Input: part model. Units: mm. Frame: model coordinates. A direction names the side the tool comes from. Round coordinates to 2 decimals unless told otherwise and drop trailing zeros. Order: outer loops, then holes, each group sorted by start corner. A loop starts at its lowest first (then second) coordinate and runs counter-clockwise, first axis right, second up. Notation, with made-up numbers: (76.5, 27) -> (94.5, 27) arc R14 ccw to (94.5, 34) -> close; hole circle Ø9 at (55.5, 30.25). An arc over 180 degrees is marked (long way). Use a Markdown table: item, result.
from build123d import *

# Parameters (mm, degrees)
SKETCH1_W                                       = 15
SKETCH1_H                                       = 24
BOSS_EXTRUDE1_DEPTH                             = 3
SKETCH2_W                                       = 8
SKETCH2_H                                       = 5
BOSS_EXTRUDE2_DEPTH                             = 6
CSK_FOR_M2_FLAT_HEAD_MACHINE_SCREW1_D           = 2.4
CSK_FOR_M2_FLAT_HEAD_MACHINE_SCREW1_CSINK_D     = 4.4
CSK_FOR_M2_FLAT_HEAD_MACHINE_SCREW1_CSINK_ANGLE = 90
FILLET1_R                                       = 2
SKETCH5_R                                       = 1.5
CUT_EXTRUDE1_DEPTH                              = 3
FILLET2_R                                       = 4


with BuildPart() as part:
    # Sketch1 → Boss-Extrude1 (new body)
    with BuildSketch(Plane.XY):
        Rectangle(SKETCH1_W, SKETCH1_H)
    extrude(amount=BOSS_EXTRUDE1_DEPTH)

    # Sketch2 → Boss-Extrude2 (add)
    with BuildSketch(Plane.XY.offset(3)):
        with Locations((0, -9.5)):
            Rectangle(SKETCH2_W, SKETCH2_H)
    extrude(amount=BOSS_EXTRUDE2_DEPTH)

    # CSK for M2 Flat Head Machine Screw1 (through all)
    with Locations(Plane(origin=(0, -7, 6), x_dir=(0, 0, 1), z_dir=(0, 1, 0))):
        with Locations((0, 0)):
            CounterSinkHole(CSK_FOR_M2_FLAT_HEAD_MACHINE_SCREW1_D / 2, CSK_FOR_M2_FLAT_HEAD_MACHINE_SCREW1_CSINK_D / 2, counter_sink_angle=CSK_FOR_M2_FLAT_HEAD_MACHINE_SCREW1_CSINK_ANGLE)

    # Fillet1
    fillet1_edges = [part.edges().sort_by_distance(p)[0] for p in [
        (-4, -9.5, 9),
        (4, -9.5, 9),
    ]]
    fillet(fillet1_edges, radius=FILLET1_R)

    # Sketch5 → Cut-Extrude1 (cut)
    with BuildSketch(Plane(origin=(0, 0, 0), x_dir=(-1, 0, 0), z_dir=(0, 0, -1))):
        with Locations((0, 5.5)):
            Circle(SKETCH5_R)
    extrude(amount=-CUT_EXTRUDE1_DEPTH, mode=Mode.SUBTRACT)

    # Fillet2
    fillet2_edges = [part.edges().sort_by_distance(p)[0] for p in [
        (-7.5, 12, 1.5),
        (7.5, 12, 1.5),
    ]]
    fillet(fillet2_edges, radius=FILLET2_R)


solid = part.part
1) Ray query, probe 1 along Z at (x, y) = (0, -10.5); probe 2 along X at (y, z) = (-10.3, 6); probe 3 along Y at (x, z) = (0, 1.1). Return the intervals inside material, ascending.
Answer key:
| item | result |
|---|---|
| probe 1 | z = 0 to 4.8, 7.2 to 9 |
| probe 2 | x = -4 to -1.2, 1.2 to 4 |
| probe 3 | y = -12 to 4, 7 to 12 |
2) Cut plane A-A on x = 0. Return loops of the section in (y, z).
Answer key:
| item | result |
|---|---|
| outline | (-12, 0) -> (4, 0) -> (4, 3) -> (-7, 3) -> (-7, 3.8) -> (-8, 4.8) -> (-12, 4.8) -> close; (-12, 7.2) -> (-8, 7.2) -> (-7, 8.2) -> (-7, 9) -> (-12, 9) -> close; (7, 0) -> (12, 0) -> (12, 3) -> (7, 3) -> close |
3) Cut plane C-C on z = 6. Return loops of the section in (x, y).
Answer key:
| item | result |
|---|---|
| outline | (-4, -12) -> (-1.2, -12) -> (-1.2, -8) -> (-2.2, -7) -> (-4, -7) -> close; (1.2, -12) -> (4, -12) -> (4, -7) -> (2.2, -7) -> (1.2, -8) -> close |
4) Draft query along X for faces 1 (the face through (-3.43, -9.46, 8.4)), 2 (the face through (0, -9, 9)), 3 (the face through (0.05, -10.03, 7.2)), 4 (the face through (6.359, 10.797, 1.521)). Return one class per face: released by +X, released by -X, zero draft, split by the parting line, or undercut.
Answer key:
| item | result |
|---|---|
| face 1 | released by -X |
| face 2 | zero draft |
| face 3 | undercut |
| face 4 | released by +X |
5) Contact query for flat-ended pins moving along their axis: P1, Ø2, axis at x = -3.5, y = 6.5, coming from the -Z side; P2, Ø1, axis at x = -5, z = 7.5, coming from the -Y side; P3, Ø1.2, axis at y = -10.5, z = 6, coming from the +X side; P4, Ø4.5, axis at x = 0, y = 5, coming from the +Z side. Output: stop coordinate, or through.
Answer key:
| item | result |
|---|---|
| P1 | stops at z = 0 |
| P2 | passes through |
| P3 | stops at x = 4 |
| P4 | stops at z = 3 |
6) Cut plane B-B on y = 5.5. Return loops of the section in (x, z).
Answer key:
| item | result |
|---|---|
| outline | (-7.5, 0) -> (-1.5, 0) -> (-1.5, 3) -> (-7.5, 3) -> close; (1.5, 0) -> (7.5, 0) -> (7.5, 3) -> (1.5, 3) -> close |
7) Set-up query: faces 5 (the face through (-4, -10, 5)), 6 (the face through (-0.1, -7, 3.3)), 7 (the face through (0, 12, 1)), 8 (the face through (4, -10, 5)), 9 (the face through (-6.359, 10.797, 1.521)). Return all of +Z, -Z, +X, -X, +Y, -Y with unobstructed straight access to the full face (end or side cutting, diameter ignored); none if empty.
Answer key:
| item | result |
|---|---|
| face 5 | +Z, -X, +Y, -Y |
| face 6 | +Z, +X, -X, +Y |
| face 7 | +Z, -Z, +X, -X, +Y |
| face 8 | +Z, +X, +Y, -Y |
| face 9 | +Z, -Z, -X, +Y |
8) Cut plane D-D on z = 1. Return loops of the section in (x, y), and give its area (3 significant figures).
Answer key:
| item | result |
|---|---|
| outline | (-7.5, -12) -> (7.5, -12) -> (7.5, 8) arc R4 ccw to (3.5, 12) -> (-3.5, 12) arc R4 ccw to (-7.5, 8) -> close; hole circle Ø3 at (0, 5.5) |
| area | 346 mm^2 |
